Could you check a few things on this model? Use its own coordinates, in mm. A direction names the side the tool comes from. Coordinates: 2 decimals unless noted, no trailing zeros. Order: outer loops, then holes, each group sorted by start corner. A loop starts at its lowest first (then second) coordinate and runs counter-clockwise, first axis right, second up. Notation, with made-up numbers: M 86.25,2.25 L 140.25,2.25 A12 ccw 140.25,20.25 Z; hole C 35.5,-23 d5. An arc over 180 degrees is marked long. One line per question, with ' | ' between items. Start each with the question number.
from build123d import *

# Parameters (mm, degrees)
F0_R     = 46.35
F1_DEPTH = 5
F2_R     = 40.9537225283
F2_W     = 20
F2_H     = 50
F3_DEPTH = 4
F5_DEPTH = 2
F6_DEPTH = 2


# Not quite as in the source:
# - a feature names something its author has since deleted; it is built from what else it names


with BuildPart() as f1:
    # F0 (on Top) → F1 (new body)
    with BuildSketch(Plane.XY):
        Circle(F0_R)
    extrude(amount=F1_DEPTH)

    # F2 (on face) → F3 (cut)
    with BuildSketch(Plane.XY.offset(5)):
        Circle(F2_R)
        Rectangle(F2_W, F2_H, mode=Mode.SUBTRACT)
    extrude(amount=-F3_DEPTH, mode=Mode.SUBTRACT)

    # F4 (on face) → F5 (join)
    with BuildSketch(Plane.XY):
        with BuildLine():
            Line((10, 45.2583970109), (10, 56.35))
            Line((10, 56.35), (0, 56.35))
            Line((0, 56.35), (-10, 56.35))
            Line((-10, 56.35), (-10, 45.2583970109))
            ThreePointArc((-10, 45.2583970109), (0, 46.35), (10, 45.2583970109))
        make_face()
    extrude(amount=F5_DEPTH)

    # F4 (on face) → F6 (join)
    with BuildSketch(Plane.XY):
        with BuildLine():
            Line((10, -56.35), (10, -45.2583970109))
            ThreePointArc((10, -45.2583970109), (0, -46.35), (-10, -45.2583970109))
            Line((-10, -45.2583970109), (-10, -56.35))
            Line((-10, -56.35), (10, -56.35))
        make_face()
    extrude(amount=F6_DEPTH)


solid = f1.part
(1) Imagine slicing it at B-B, the plane x = 0. Write out the boundary of the cut face in (y, z), plus the area to 3 significant figures.
(2) Imagine slicing it at D-D, the plane x = -12. Write out the boundary of the cut face in (y, z), plus the area to 3 significant figures.
(3) Imagine slicing it at C-C, the plane y = 0. Write out the boundary of the cut face in (x, z), plus the area to 3 significant figures.
(4) On a 3-axis mill with a long thin cutter (end or side, diameter ignored), from which of +Z, -Z, +X, -X, +Y, -Y can I reach the whole of each face in a straight line? I mean faces 1 (the flat face through (-10, 0, 3)), 2 (the flat face through (-1, 1, 0)). Say none if no direction works.
(5) We'd pull the mould along X, two halves only. Please class faces 3 (the flat face through (0, -51, 2)), 4 (the flat face through (18, 1, 1)), 5 (the cylindrical face through (-10.048, -45.248, 2.465)): +X half, -X half, draft (parallel to the pull), parting line (faces both ways), or undercut.
(6) For P1, Ø3.5, axis at x = -5, y = -49, coming from the +Z side; P2, Ø2, axis at y = 13, z = 4, coming from the +X side; P3, Ø0.6, axis at y = 51.5, z = 1, coming from the +X side, each with a flat end and sliding along its axis, tell me the tip position at first contact or that it passes through.
(7) If I drill on line 1 along Y through (x, z) = (0, 2.1); line 2 along X through (y, z) = (13.5, 1.65); line 3 along X through (y, z) = (22.5, 3.2), over which ranges is the centre line in solid material (lowest first)? Write a range as from..to.
(8) Imagine slicing it at A-A, the plane z = 3.45. Write out the boundary of the cut face in (x, y).
Answers:
1) outline: M -56.35,0 L 56.35,0 L 56.35,2 L 46.35,2 L 46.35,5 L 40.95,5 L 40.95,1 L 25,1 L 25,5 L -25,5 L -25,1 L -40.95,1 L -40.95,5 L -46.35,5 L -46.35,2 L -56.35,2 Z | area: 376 mm²
2) outline: M -44.77,0 L 44.77,0 L 44.77,5 L 39.16,5 L 39.16,1 L -39.16,1 L -39.16,5 L -44.77,5 Z | area: 134 mm²
3) outline: M -46.35,0 L 46.35,0 L 46.35,5 L 40.95,5 L 40.95,1 L 10,1 L 10,5 L -10,5 L -10,1 L -40.95,1 L -40.95,5 L -46.35,5 Z | area: 216 mm²
4) face 1: +Z | face 2: -Z, +X, -X, +Y, -Y
5) face 3: draft | face 4: undercut | face 5: parting line
6) P1: z = 2 | P2: x = 44.77 | P3: x = 10
7) line 1: -46.35..-40.95, -25..25, 40.95..46.35 | line 2: -44.34..-38.66, -10..10, 38.66..44.34 | line 3: -40.52..-34.22, -10..10, 34.22..40.52
8) outline: C 0,0 d92.7; M -10,-25 L 10,-25 L 10,25 L -10,25 Z; hole C 0,0 d81.91
